Could you check a few things on this drawing? It's one solid part, dimensions in mm from its lowest x, y, z. A direction names the side the tool comes from. Give positions to 0.01 mm unless a question says otherwise; leave off trailing zeros. Loops run counter-clockwise (first coordinate to the right, second up) from the corner with the lowest first, then second, coordinate; pieces in that order, holes last. Notation, with made-up numbers: M -1,-32.5 L 55,-32.5 A11 cw 55,-26.5 Z; hole C 56,70 d4. An arc over 180 degrees is marked long. One line per item, written item: value. Start each with the question number.
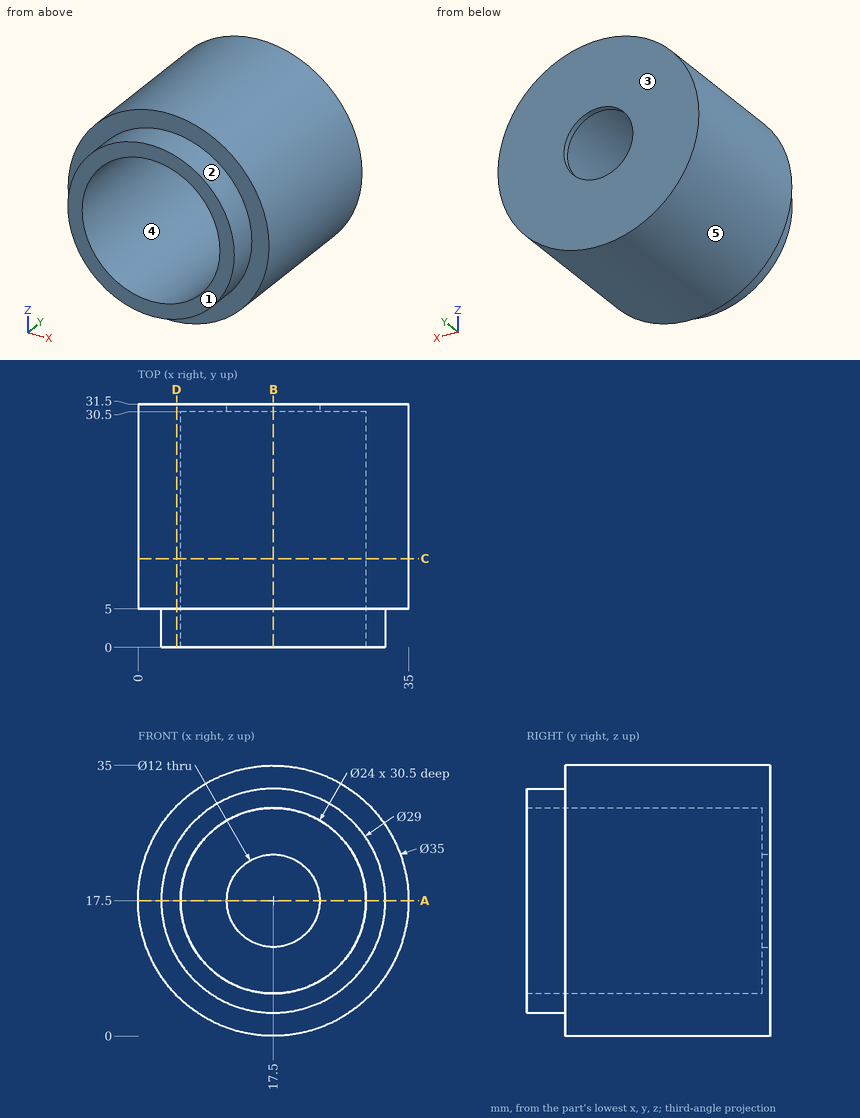
Q1. I need wall thicknesses on line 1 along Z through (x, y) = (17.5, 31.1); line 2 along Z through (x, y) = (17, 30). Which ranges of each line are inside material? Lowest first, please.
Q2. If we section it at C-C, the plane y = 11.5: Write out the boundary of the cut face in (x, z).
Q3. If we section it at A-A, the plane z = 17.5: Write out the boundary of the cut face in (x, y), plus the area to 4 significant figures.
Q4. If we section it at D-D, the plane x = 5: Write out the boundary of the cut face in (y, z).
Q5. If we section it at B-B, the plane x = 17.5: Write out the boundary of the cut face in (y, z), plus the area to 4 significant figures.
Q6. For P1, Ø4, axis at x = 18.5, y = 21.5, coming from the -Z side; P2, Ø10, axis at x = 9.5, y = 24, coming from the -Z side; P3, Ø3, axis at x = 25, z = 24, coming from the -Y side; P4, Ø10, axis at x = 30, y = 22, coming from the +Z side, each with a flat end and sliding along its axis, tell me the tip position at first contact or that it passes through.
Q7. Which directions (+Z, -Z, +X, -X, +Y, -Y) give clear straight access to the entire face, cutting with the end or side of a thin tool? Please do the marked faces 1 and 2.
Q8. If we mould it in two halves opening along X, with no side actions, what happens to the marked faces 3, 4 and 5? For each: released by +X, released by -X, zero draft, split by the parting line, or undercut.
Response:
1. line 1: 0 to 11.5, 23.5 to 35
1. line 2: 0.01 to 5.51, 29.49 to 34.99
2. outline: C 17.5,17.5 d35; hole C 17.5,17.5 d24
3. outline: M 0,5 L 3,5 L 3,0 L 5.5,0 L 5.5,30.5 L 11.5,30.5 L 11.5,31.5 L 0,31.5 Z; M 23.5,30.5 L 29.5,30.5 L 29.5,0 L 32,0 L 32,5 L 35,5 L 35,31.5 L 23.5,31.5 Z
3. area: 328.5 mm^2
4. outline: M 0,10.15 L 5,10.15 L 5,5.25 L 31.5,5.25 L 31.5,29.75 L 5,29.75 L 5,24.85 L 0,24.85 Z
5. outline: M 0,3 L 5,3 L 5,0 L 31.5,0 L 31.5,11.5 L 30.5,11.5 L 30.5,5.5 L 0,5.5 Z; M 0,29.5 L 30.5,29.5 L 30.5,23.5 L 31.5,23.5 L 31.5,35 L 5,35 L 5,32 L 0,32 Z
5. area: 328.5 mm^2
6. P1: z = 0
6. P2: z = 0.26
6. P3: y = 30.5
6. P4: z = 33.31
7. face 1: +Z, -Z, +X, -X, -Y
7. face 2: -Y
8. face 3: zero draft
8. face 4: undercut
8. face 5: split by the parting line
